The model under review builds one solid part; all positions refer to its coordinate system, in mm. Round coordinates to 2 decimals unless told otherwise and drop trailing zeros. Order: outer loops, then holes, each group sorted by start corner. A loop starts at its lowest first (then second) coordinate and runs counter-clockwise, first axis right, second up.
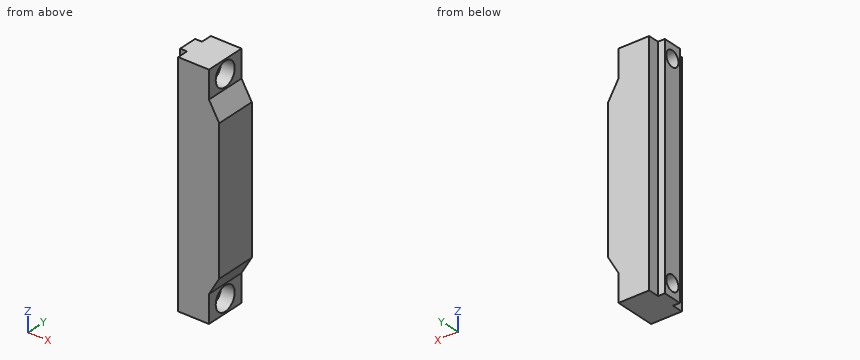
```python
from build123d import *

# Parameters (mm, degrees)
BOSS_EXTRUDE1_DEPTH = 9.525
BOSS_EXTRUDE2_START = -12.7
SKETCH2_W           = 107.95
SKETCH2_H           = 8.7376
BOSS_EXTRUDE2_DEPTH = 3.175
CUT_EXTRUDE2_START  = 4.7498
SKETCH3_R           = 3.5687
CUT_EXTRUDE2_DEPTH  = 22.225
CUT_EXTRUDE4_START  = 4.7498
SKETCH4_R           = 5.5626
CUT_EXTRUDE4_DEPTH  = 6.35


with BuildPart() as part:
    # Sketch1 → Boss-Extrude1 (new, symmetric)
    with BuildSketch(Plane(origin=(0, 0, 0), x_dir=(1, 0, 0), z_dir=(0, 1, 0))):
        Polygon((-9.525, -53.975), (-9.525, 53.975), (4.7498, 53.975), (4.7498, 41.275), (9.525, 33.004110984), (9.525, -33.004110984), (4.7498, -41.275), (4.7498, -53.975), align=None)
    extrude(amount=BOSS_EXTRUDE1_DEPTH, both=True)

    # Sketch2 → Boss-Extrude2 (add)
    with BuildSketch(Plane(origin=(0, 0, 0), x_dir=(0, 0, -1), z_dir=(1, 0, 0)).offset(BOSS_EXTRUDE2_START)):
        Rectangle(SKETCH2_W, SKETCH2_H)
    extrude(amount=BOSS_EXTRUDE2_DEPTH)

    # Sketch3 → Cut-Extrude2 (cut)
    with BuildSketch(Plane(origin=(0, 0, 0), x_dir=(0, 0, -1), z_dir=(1, 0, 0)).offset(CUT_EXTRUDE2_START)):
        with Locations((-47.625, 0)):
            Circle(SKETCH3_R)
        with Locations((47.625, 0)):
            Circle(SKETCH3_R)
    extrude(amount=-CUT_EXTRUDE2_DEPTH, mode=Mode.SUBTRACT)

    # Sketch4 → Cut-Extrude4 (cut)
    with BuildSketch(Plane(origin=(0, 0, 0), x_dir=(0, 0, -1), z_dir=(1, 0, 0)).offset(CUT_EXTRUDE4_START)):
        with Locations((-47.625, 0)):
            Circle(SKETCH4_R)
        with Locations((47.625, 0)):
            Circle(SKETCH4_R)
    extrude(amount=-CUT_EXTRUDE4_DEPTH, mode=Mode.SUBTRACT)


solid = part.part
```
(1) Consider section B-B (x = 2.75). Write out the cut boundary in (y, z) (3 decimals).
Data:
outline: (-9.525, -53.975) - (9.525, -53.975) - (9.525, 53.975) - (-9.525, 53.975) - close; hole circle Ø11.125 at (0, -47.625); hole circle Ø11.125 at (0, 47.625)
(2) Consider section A-A (y = 0). Write out the cut boundary in (x, z) (3 decimals).
Data:
outline: (-12.7, -53.975) - (4.75, -53.975) - (4.75, -53.188) - (-1.6, -53.188) - (-1.6, -51.194) - (-12.7, -51.194) - close; (-12.7, -44.056) - (-1.6, -44.056) - (-1.6, -42.062) - (4.75, -42.062) - (4.75, -41.275) - (9.525, -33.004) - (9.525, 33.004) - (4.75, 41.275) - (4.75, 42.062) - (-1.6, 42.062) - (-1.6, 44.056) - (-12.7, 44.056) - close; (-12.7, 51.194) - (-1.6, 51.194) - (-1.6, 53.188) - (4.75, 53.188) - (4.75, 53.975) - (-12.7, 53.975) - close
(3) Insertion check: pin 1 (1.5 mm diameter, centred on x = -10, z = -28.5, fed in from +Y) (3 decimals); pin 2 (2.5 mm diameter, centred on x = -11, z = 4, fed in from -Y); pin 3 (6.5 mm diameter, centred on y = -3.5, z = 46.5, fed in from +X); pin 4 (4 mm diameter, centred on y = 6.5, z = 29, fed in from -X) (3 decimals). Each pin has a flat end and moves straight along its axis. Give the tip position at first contact, or say it passes through.
Data:
pin 1: stops at y = 9.525
pin 2: stops at y = -4.37
pin 3: stops at x = 4.75
pin 4: stops at x = -9.525
(4) To check wall thickness, follow probe 1 along Z at (x, y) = (-0.5, 0.5) (3 decimals); probe 2 along Z at (x, y) = (3.5, -2.5) (3 decimals); probe 3 along X at (y, z) = (4.5, 0) (3 decimals). State the ranges of each line that lie inside material, in increasing order.
Data:
probe 1: z = -53.975 to -53.165, -42.085 to 42.085, 53.165 to 53.975
probe 2: z = -53.975 to -52.594, -42.656 to 42.656, 52.594 to 53.975
probe 3: x = -9.525 to 9.525
(5) Consider section D-D (z = 10). Write out the cut boundary in (x, y) (3 decimals).
Data:
outline: (-12.7, -4.369) - (-9.525, -4.369) - (-9.525, -9.525) - (9.525, -9.525) - (9.525, 9.525) - (-9.525, 9.525) - (-9.525, 4.369) - (-12.7, 4.369) - close
(6) Consider section C-C (z = -46). Write out the cut boundary in (x, y) (3 decimals), and give its area (3 significant figures).
Data:
outline: (-12.7, -4.369) - (-9.525, -4.369) - (-9.525, -9.525) - (4.75, -9.525) - (4.75, -5.32) - (-1.6, -5.32) - (-1.6, -3.177) - (-12.7, -3.177) - close; (-12.7, 3.177) - (-1.6, 3.177) - (-1.6, 5.32) - (4.75, 5.32) - (4.75, 9.525) - (-9.525, 9.525) - (-9.525, 4.369) - (-12.7, 4.369) - close
area: 162 mm2
